from build123d import *

# Parameters (mm, degrees)
SKETCH1_W           = 45
SKETCH1_H           = 115
BOSS_EXTRUDE1_DEPTH = 23
SKETCH2_R           = 33.5
CUT_EXTRUDE1_DEPTH  = 121
SKETCH3_W           = 10
SKETCH3_H           = 10
CUT_EXTRUDE3_DEPTH  = 31
FILLET2_R           = 3
FILLET3_R           = 3
SKETCH5_W           = 15
SKETCH5_H           = 1.5
SKETCH5_W_2         = 1.5
SKETCH5_H_2         = 12.5
SKETCH5_H_3         = 19.25
CUT_EXTRUDE4_DEPTH  = 3


with BuildPart() as part:
    # Sketch1 → Boss-Extrude1 (new body)
    with BuildSketch(Plane(origin=(0, 0, 0), x_dir=(0, 0, -1), z_dir=(1, 0, 0))):
        Rectangle(SKETCH1_W, SKETCH1_H)
    extrude(amount=BOSS_EXTRUDE1_DEPTH)

    # Sketch2 → Cut-Extrude1 (cut)
    with BuildSketch(Plane(origin=(0, 57.5, 0), x_dir=(1, 0, 0), z_dir=(0, 1, 0))):
        with Locations((47.819347292, 0)):
            Circle(SKETCH2_R)
    extrude(amount=-CUT_EXTRUDE1_DEPTH, mode=Mode.SUBTRACT)

    # Sketch3 → Cut-Extrude3 (cut)
    with BuildSketch(Plane.ZY):
        with Locations((12.5, -47.5)):
            Rectangle(SKETCH3_W, SKETCH3_H)
        with Locations((-12.5, -47.5)):
            Rectangle(SKETCH3_W, SKETCH3_H)
        with Locations((0, -22.5)):
            Rectangle(SKETCH3_W, SKETCH3_H)
        Rectangle(SKETCH3_W, SKETCH3_H)
        with Locations((0, 22.5)):
            Rectangle(SKETCH3_W, SKETCH3_H)
        with Locations((12.5, 47.5)):
            Rectangle(SKETCH3_W, SKETCH3_H)
        with Locations((-12.5, 47.5)):
            Rectangle(SKETCH3_W, SKETCH3_H)
    extrude(amount=-CUT_EXTRUDE3_DEPTH, mode=Mode.SUBTRACT)

    # Fillet2
    fillet2_edges = [part.edges().sort_by_distance(p)[0] for p in [
        (9.626816789, -42.5, 17.5),
        (9.626816789, -52.5, 17.5),
        (7.584845929, -42.5, 7.5),
        (7.584845929, 52.5, -7.5),
        (7.584845929, 42.5, -7.5),
        (9.626816789, 42.5, -17.5),
        (9.626816789, 52.5, -17.5),
        (9.626816789, 52.5, 17.5),
        (9.626816789, 42.5, 17.5),
        (7.584845929, 42.5, 7.5),
        (7.584845929, 52.5, 7.5),
        (7.347291571, 27.5, 5),
        (7.347291571, 17.5, 5),
        (7.347291571, 17.5, -5),
        (7.347291571, 27.5, -5),
        (7.347291571, 5, 5),
        (7.347291571, -5, 5),
        (7.347291571, -5, -5),
        (7.347291571, 5, -5),
        (7.347291571, -17.5, 5),
        (7.347291571, -27.5, 5),
        (7.347291571, -27.5, -5),
        (7.347291571, -17.5, -5),
        (7.584845929, -42.5, -7.5),
        (7.584845929, -52.5, -7.5),
        (9.626816789, -52.5, -17.5),
        (9.626816789, -42.5, -17.5),
    ]]
    fillet(fillet2_edges, radius=FILLET2_R)

    # Fillet3
    fillet3_edges = [part.edges().sort_by_distance(p)[0] for p in [
        (7.584845929, -52.5, 7.5),
    ]]
    fillet(fillet3_edges, radius=FILLET3_R)

    # Sketch5 → Cut-Extrude4 (cut)
    with BuildSketch(Plane.ZY):
        with Locations((0, -47.5)):
            Rectangle(SKETCH5_W, SKETCH5_H)
        with Locations((0, -11.25)):
            Rectangle(SKETCH5_W_2, SKETCH5_H_2)
        with Locations((0, -37.125)):
            Rectangle(SKETCH5_W_2, SKETCH5_H_3)
        with Locations((0, 11.25)):
            Rectangle(SKETCH5_W_2, SKETCH5_H_2)
        with Locations((0, 37.125)):
            Rectangle(SKETCH5_W_2, SKETCH5_H_3)
        with Locations((0, 47.5)):
            Rectangle(SKETCH5_W, SKETCH5_H)
    extrude(amount=-CUT_EXTRUDE4_DEPTH, mode=Mode.SUBTRACT)


solid = part.part
The model under review builds one solid part; all positions refer to its coordinate system, in mm. A direction names the side the tool comes from. Round coordinates to 2 decimals unless told otherwise and drop trailing zeros. Loops run counter-clockwise (first coordinate to the right, second up) from the corner with the lowest first, then second, coordinate; pieces in that order, holes last. Notation, with made-up numbers: (76.5, -16.5) - (127.5, -16.5) arc R17 ccw to (127.5, -2.5) - close; hole circle Ø9 at (44.5, 30). An arc over 180 degrees is marked (long way). Use CSV: the item, a comma, the result in double quotes.
(1) Machinability: for faces 1 (the cylindrical face through (8.12, -43.36, -8.4)), 2 (the flat face through (1, -46.75, -4)), which of the approach directions +Z, -Z, +X, -X, +Y, -Y give a long, thin tool a straight path to every point of the face, cutting with its end or side? Answer none if there is none.
Working result:
face 1,"+X, -X"
face 2,"-X"
(2) Take a section at A-A, the plane y = -0.5. Give the boundary of the cut face in (x, z).
Working result:
outline,"(0, -22.5) - (23, -22.5) arc R33.5 cw to (14.69, -5) - (0, -5) - close; (0, 5) - (14.69, 5) arc R33.5 cw to (23, 22.5) - (0, 22.5) - close"
(3) Take a section at C-C, the plane z = 19. Give the boundary of the cut face in (x, y), plus the area to 3 significant figures.
Working result:
outline,"(0, -57.5) - (20.23, -57.5) - (20.23, 57.5) - (0, 57.5) - close"
area,"2,330 mm^2"
(4) Take a section at B-B, the plane x = 4.75. State how many separate pieces and enclosed holes the cut face has, plus the area to 3 significant figures.
Working result:
separate pieces,"1"
enclosed holes,"7"
area,"4,530 mm^2"
(5) For line 1 (Y direction, x = 3.5, z = -13.5); line 2 (Y direction, x = 13.75, z = 1); line 3 (Z direction, x = 12.25, y = -49), list the stretches that pass through material, from the lowest coordinate up.
Working result:
line 1,"y = -57.5 to -52.5, -42.5 to 42.5, 52.5 to 57.5"
line 2,"y = -57.5 to -27.5, -17.5 to -5, 5 to 17.5, 27.5 to 57.5"
line 3,"z = -22.5 to -17.5, -7.5 to 7.5, 17.5 to 22.5"
